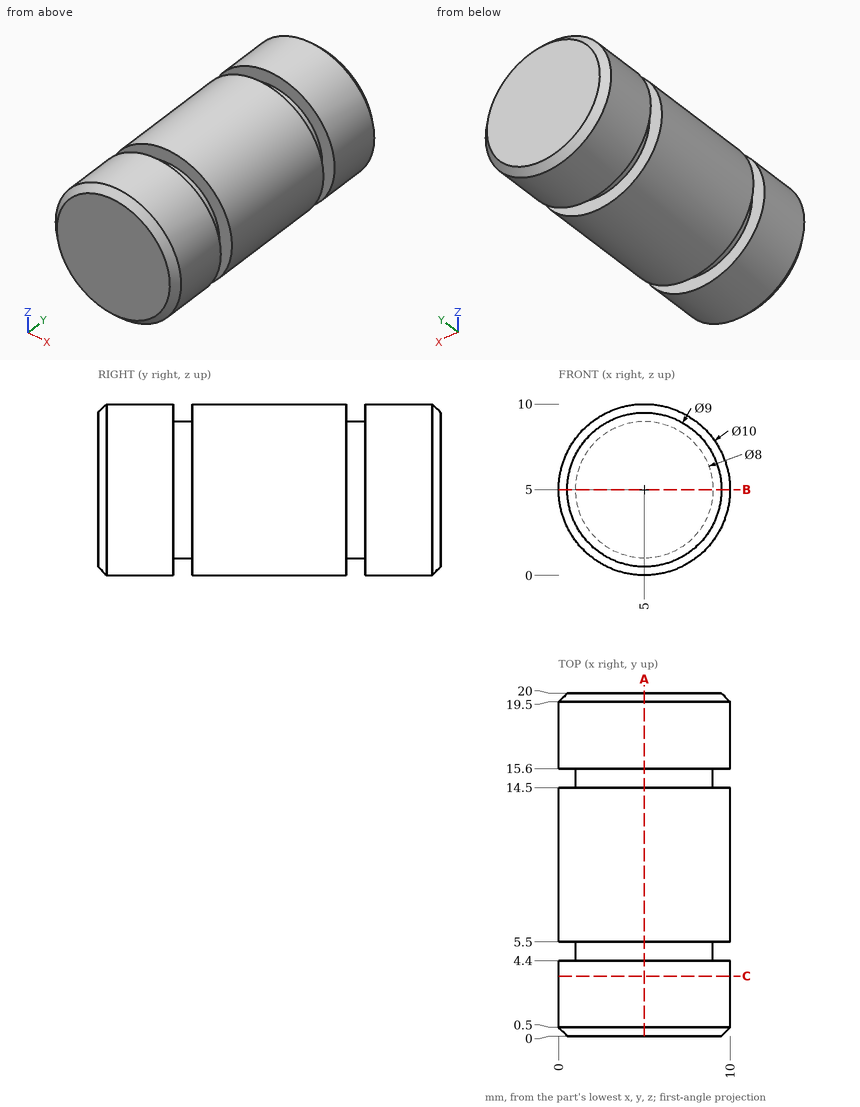
Source: three-view drawing plus pictorial views. Frame: mm from the lowest corner of the part. Round coordinates to 2 decimals unless told otherwise and drop trailing zeros. Loops run counter-clockwise (first coordinate to the right, second up) from the corner with the lowest first, then second, coordinate; pieces in that order, holes last. Notation, with made-up numbers: M 29.5,-28.5 L 64.5,-28.5 A31 cw 64.5,4.5 Z; hole C 13.5,69.25 d2. An arc over 180 degrees is marked long. Answer as CSV lines item,"result". Start each with the question number.
(1) First-contact query: pin 1 (1 mm diameter, centred on x = 7.5, y = 4.5, fed in from -Z); pin 2 (3 mm diameter, centred on x = 4.5, z = 7, fed in from -Y); pin 3 (3 mm diameter, centred on x = 1, y = 13, fed in from +Z); pin 4 (4 mm diameter, centred on y = 15, z = 8, fed in from -X). Flat tips, straight axial feed; report the tip coordinate or a pass-through.
(2) Section C-C, the plane y = 3.5. Output: boundary loops of the cut face in (x, z), plus the area to 3 significant figures.
(3) Section A-A, the plane x = 5. Output: boundary loops of the cut face in (y, z).
(4) Line query: line 1 (Y direction, x = 4, z = 1); line 2 (Y direction, x = 1.5, z = 8.5); line 3 (X direction, y = 9, z = 8). Output: solid intervals per line, ascending. Write a range as [from, to].
(5) Section B-B, the plane z = 5. Output: boundary loops of the cut face in (x, y).
Values found:
1,pin 1,"stops at z = 0.42"
1,pin 2,"stops at y = 0"
1,pin 3,"stops at z = 9.33"
1,pin 4,"stops at x = 0.11"
2,outline,"C 5,5 d10"
2,area,"78.5 mm²"
3,outline,"M 0,0.5 L 0.5,0 L 4.4,0 L 4.4,1 L 5.5,1 L 5.5,0 L 14.5,0 L 14.5,1 L 15.6,1 L 15.6,0 L 19.5,0 L 20,0.5 L 20,9.5 L 19.5,10 L 15.6,10 L 15.6,9 L 14.5,9 L 14.5,10 L 5.5,10 L 5.5,9 L 4.4,9 L 4.4,10 L 0.5,10 L 0,9.5 Z"
4,line 1,"y = [0, 4.4], [5.5, 14.5], [15.6, 20]"
4,line 2,"y = [0.45, 4.4], [5.5, 14.5], [15.6, 19.55]"
4,line 3,"x = [1, 9]"
5,outline,"M 0,0.5 L 0.5,0 L 9.5,0 L 10,0.5 L 10,4.4 L 9,4.4 L 9,5.5 L 10,5.5 L 10,14.5 L 9,14.5 L 9,15.6 L 10,15.6 L 10,19.5 L 9.5,20 L 0.5,20 L 0,19.5 L 0,15.6 L 1,15.6 L 1,14.5 L 0,14.5 L 0,5.5 L 1,5.5 L 1,4.4 L 0,4.4 Z"
